from build123d import *

# Parameters (mm, degrees)
SKETCH1_W           = 200
SKETCH1_H           = 200
BOSS_EXTRUDE1_DEPTH = 25
SKETCH2_W           = 200
SKETCH2_H           = 200
BOSS_EXTRUDE2_DEPTH = 50


with BuildPart() as part:
    # Sketch1 → Boss-Extrude1 (new body)
    with BuildSketch(Plane.XY):
        Rectangle(SKETCH1_W, SKETCH1_H)
    extrude(amount=BOSS_EXTRUDE1_DEPTH)

    # Sketch2 → Boss-Extrude2 (add)
    with BuildSketch(Plane(origin=(0, 0, 0), x_dir=(-1, 0, 0), z_dir=(0, 0, -1))):
        with Locations((0, 200)):
            Rectangle(SKETCH2_W, SKETCH2_H)
    extrude(amount=-BOSS_EXTRUDE2_DEPTH)


solid = part.part
Can you work these out from the model? Positions are in its coordinate system, mm. A direction names the side the tool comes from. Give positions to 0.01 mm unless a question says otherwise; leave off trailing zeros. Order: outer loops, then holes, each group sorted by start corner. A loop starts at its lowest first (then second) coordinate and runs counter-clockwise, first axis right, second up. Notation, with made-up numbers: M -7.5,15 L 10.5,15 A22 cw 10.5,25 Z; hole C 24,89.5 d8. An arc over 180 degrees is marked long. One line per question, with ' | ' between items.
Item 1: Please list where these lines run through material, in increasing order: L1, parallel to Z at x = -47, y = 4.5; L2, parallel to Y at x = 14.5, z = 44.5.
Answer block:
L1: z = 0 to 25 | L2: y = 100 to 300
Item 2: Suppose I cut it at A-A, the plane y = -26.5. Write out the boundary of the cut face in (x, z), then the cut area to 3 significant figures.
Answer block:
outline: M -100,0 L 100,0 L 100,25 L -100,25 Z | area: 5,000 mm2
Item 3: I'm going to push flat-ended pins straight in: pin 1 Ø3 at (x, y) = (-36.5, 40) entering from +Z; pin 2 Ø6 at (x, z) = (-30.5, 30) entering from -Y. Where does each tip first touch, or does it pass through?
Answer block:
pin 1: stops at z = 25 | pin 2: stops at y = 100
Item 4: For faces 1 (the face through (100, 142, 19)), 2 (the face through (1, 100, 37)), which set-ups out of +Z, -Z, +X, -X, +Y, -Y let a thin tool reach every point of the face, with its end or its side?
Answer block:
face 1: +Z, -Z, +X, +Y, -Y | face 2: +Z, +X, -X, -Y
Item 5: Suppose I cut it at B-B, the plane z = 33. Write out the boundary of the cut face in (x, y).
Answer block:
outline: M -100,100 L 100,100 L 100,300 L -100,300 Z
Item 6: Suppose I cut it at C-C, the plane x = 52.5. Write out the boundary of the cut face in (y, z).
Answer block:
outline: M -100,0 L 300,0 L 300,50 L 100,50 L 100,25 L -100,25 Z
